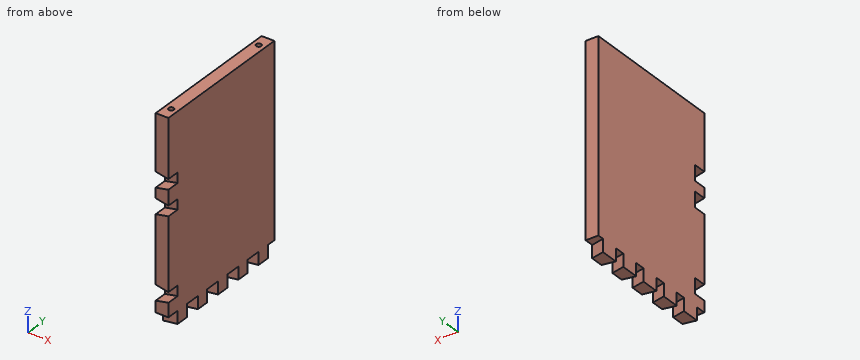
```python
from build123d import *

# Parameters (mm, degrees)
F0_W     = 115
F0_H     = 160
F1_DEPTH = 10
F3_DEPTH = 10
F5_DEPTH = 10
F6_R     = 2
F7_DEPTH = 10


with BuildPart() as f1:
    # F0 (on Right) → F1 (new body)
    with BuildSketch(Plane.YZ):
        with Locations((22.5, 7.532959)):
            Rectangle(F0_W, F0_H)
    extrude(amount=F1_DEPTH)

    # F2 (on face) → F3 (cut)
    with BuildSketch(Plane.XZ.offset(35)):
        Polygon((10, 41.532959), (0, 43.532959), (0, 31.532959), (10, 33.532959), align=None)
        Polygon((10, 21.532959), (0, 23.532959), (0, 11.532959), (10, 13.532959), align=None)
        Polygon((10, -43.467041), (0, -41.467041), (0, -53.467041), (10, -51.467041), align=None)
    extrude(amount=-F3_DEPTH, mode=Mode.SUBTRACT)

    # F4 (on face) → F5 (cut)
    with BuildSketch(Plane(origin=(0, 0, -72.467041), x_dir=(1, 0, 0), z_dir=(0, 0, -1))):
        Polygon((10, 37), (0, 35), (0, 27), (10, 25), align=None)
        Polygon((10, 3), (10, 15), (0, 13), (0, 5), align=None)
        Polygon((10, -19), (10, -7), (0, -9), (0, -17), align=None)
        Polygon((10, -41), (10, -29), (0, -31), (0, -39), align=None)
        Polygon((10, -63), (10, -51), (0, -53), (0, -61), align=None)
        Polygon((10, -85), (10, -73), (0, -75), (0, -83), align=None)
    extrude(amount=-F5_DEPTH, mode=Mode.SUBTRACT)

    # F6 (on face) → F7 (cut)
    with BuildSketch(Plane.XY.offset(87.532959)):
        with Locations((5, 70)):
            Circle(F6_R)
        with Locations((5, -25)):
            Circle(F6_R)
    extrude(amount=-F7_DEPTH, mode=Mode.SUBTRACT)


solid = f1.part
```
Part model, mm, in its own coordinate system. Coordinates: 2 decimals unless noted, no trailing zeros. Loops run counter-clockwise (first coordinate to the right, second up) from the corner with the lowest first, then second, coordinate; pieces in that order, holes last. Notation, with made-up numbers: (12, 37) - (17, 37) arc R20 ccw to (17, 47) - close; hole circle Ø11 at (-23.75, 70). An arc over 180 degrees is marked (long way). Write item = value, one per line. Start each with the question number.
Item 1: Cut at A-A, the plane y = 70. Give the cut face in (x, z), and give its area (3 significant figures).
Item 2: Flat gauge pins, fed straight in: pin 1 Ø3.5 at (x, y) = (5, 70) entering from +Z; pin 2 Ø3 at (x, y) = (4.5, -25.5) entering from +Z; pin 3 Ø3 at (x, y) = (3.5, 12) entering from -Z; pin 4 Ø3 at (x, z) = (4.5, 18) entering from -Y. Where does each tip first touch, or does it go through?
Item 3: Wall check: L1, parallel to Y at x = 5, z = 85.5; L2, parallel to Z at x = 4.25, y = 16.5. Give the ranges that are in metal, low to high. Write a range as from..to.
The answers:
q1.outline = (0, -72.47) - (10, -72.47) - (10, 87.53) - (7, 87.53) - (7, 77.53) - (3, 77.53) - (3, 87.53) - (0, 87.53) - close
q1.area = 1,560 mm2
q2.pin_1 = 77.53
q2.pin_2 = 87.53
q2.pin_3 = -62.47
q2.pin_4 = -25
q3.L1 = -35..-27, -23..68, 72..80
q3.L2 = -62.47..87.53
